Design review of the part built by this model. Coordinates are the model's own, in mm. Face numbers are marked on the shaded views. A direction names the side the tool comes from. Round coordinates to 2 decimals unless told otherwise and drop trailing zeros. Loops run counter-clockwise (first coordinate to the right, second up) from the corner with the lowest first, then second, coordinate; pieces in that order, holes last. Notation, with made-up numbers: M -14.75,85.25 L 22.25,85.25 A32 ccw 22.25,124.25 Z; hole C 16,27.25 d7. An arc over 180 degrees is marked long. Use a Markdown table: item, result.
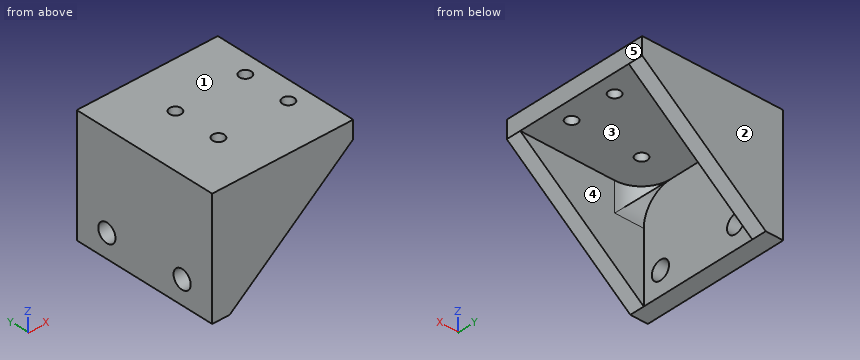
from build123d import *

# Parameters (mm, degrees)
EXTRUDE_1_DEPTH     = 12.6
SKETCH_2_W          = 21.2
SKETCH_2_H          = 20.2
CUT_EXTRUDE_1_DEPTH = 17
SKETCH_3_R          = 1
CUT_EXTRUDE_2_DEPTH = 34.828981658
SKETCH_4_R          = 1.6
CUT_EXTRUDE_3_DEPTH = 32.75216528
FILLET_1_R          = 5
CUT_EXTRUDE_4_DEPTH = 17


with BuildPart() as part:
    # 草图1 → 凸台-拉伸1 (new, symmetric)
    with BuildSketch(Plane(origin=(0, 0, 0), x_dir=(1, 0, 0), z_dir=(0, 1, 0))):
        Polygon((0, 0), (24.2, 0), (24.2, 3), (3, 20), (0, 20), align=None)
    extrude(amount=EXTRUDE_1_DEPTH, both=True)

    # 草图2 → 切除-拉伸1 (cut)
    with BuildSketch(Plane(origin=(0, 0, -20), x_dir=(-1, 0, 0), z_dir=(0, 0, -1))):
        with Locations((-13.6, 0)):
            Rectangle(SKETCH_2_W, SKETCH_2_H)
    extrude(amount=-CUT_EXTRUDE_1_DEPTH, mode=Mode.SUBTRACT)

    # 草图3 → 切除-拉伸2 (cut, through all)
    with BuildSketch(Plane.XY):
        with Locations((21, -4)):
            Circle(SKETCH_3_R)
        with Locations(Location((21, 4, 0), (0, 0, 180))):
            Circle(SKETCH_3_R)
        with Locations((9, 4)):
            Circle(SKETCH_3_R)
        with Locations(Location((9, -4, 0), (0, 0, 180))):
            Circle(SKETCH_3_R)
    extrude(amount=-CUT_EXTRUDE_2_DEPTH, mode=Mode.SUBTRACT)

    # 草图4 → 切除-拉伸3 (cut, through all)
    with BuildSketch(Plane(origin=(3, 0, 0), x_dir=(0, 0, -1), z_dir=(1, 0, 0))):
        with Locations(Location((16, 7, 0), (0, 0, 90))):
            Circle(SKETCH_4_R)
        with Locations(Location((16, -7, 0), (0, 0, 270))):
            Circle(SKETCH_4_R)
    extrude(amount=-CUT_EXTRUDE_3_DEPTH, mode=Mode.SUBTRACT)

    # 圆角1
    fillet_1_edges = [part.edges().sort_by_distance(p)[0] for p in [
        (13.6, -10.1, -3),
        (13.6, 10.1, -3),
    ]]
    fillet(fillet_1_edges, radius=FILLET_1_R)

    # 草图6 → 切除-拉伸4 (cut)
    with BuildSketch(Plane(origin=(0, 0, -20), x_dir=(-1, 0, 0), z_dir=(0, 0, -1))):
        with BuildLine():
            Line((-3, -5.1), (-3, 5.1))
            ThreePointArc((-3, 5.1), (-4.464466094, 8.635533906), (-8, 10.1))
            Line((-8, 10.1), (-24.2, 10.1))
            Line((-24.2, 10.1), (-24.2, -10.1))
            Line((-24.2, -10.1), (-8, -10.1))
            ThreePointArc((-8, -10.1), (-4.464466094, -8.635533906), (-3, -5.1))
        make_face()
    extrude(amount=-CUT_EXTRUDE_4_DEPTH, mode=Mode.SUBTRACT)


solid = part.part
1. Take a section at A-A on y = -4. Give the boundary of the cut face in (x, z), and give its area (3 significant figures).
Check values:
| item | result |
|---|---|
| outline | M 0,-20 L 3,-20 L 3,-3 L 8,-3 L 8,0 L 0,0 Z; M 10,-3 L 20,-3 L 20,0 L 10,0 Z; M 22,-3 L 24.2,-3 L 24.2,0 L 22,0 Z |
| area | 112 mm² |
2. Insertion check: pin 1 (3.5 mm diameter, centred on y = -7, z = -16, fed in from +X); pin 2 (3 mm diameter, centred on x = 9.5, y = 6.5, fed in from -Z). Each pin has a flat end and moves straight along its axis. Give the tip position at first contact, or say it passes through.
Check values:
| item | result |
|---|---|
| pin 1 | stops at x = 3 |
| pin 2 | stops at z = -3 |
3. The part is to be moulded in two halves that separate along Y. For the marked faces 1, 2 and 3, say which applies: pulls with the +Y half, pulls with the -Y half, needs draft (parallel to the pull), parting line crosses it, or undercut.
Check values:
| item | result |
|---|---|
| face 1 | needs draft |
| face 2 | pulls with the +Y half |
| face 3 | undercut |
4. Take a section at C-C on y = 7. Give the boundary of the cut face in (x, z).
Check values:
| item | result |
|---|---|
| outline | M 0,-20 L 3,-20 L 3,-17.6 L 0,-17.6 Z; M 0,-14.4 L 3,-14.4 L 3,-3.38 L 3.38,-3.38 L 3.38,-3 L 24.2,-3 L 24.2,0 L 0,0 Z |
5. Machinability: for the marked faces 4 and 5, which of the approach directions +Z, -Z, +X, -X, +Y, -Y give a long, thin tool a straight path to every point of the face, cutting with its end or side? Answer none if there is none.
Check values:
| item | result |
|---|---|
| face 4 | -Z, +X |
| face 5 | +Z, -Z, +X, +Y, -Y |
6. Take a section at B-B on x = 9. Give the boundary of the cut face in (y, z).
Check values:
| item | result |
|---|---|
| outline | M -12.6,-15.19 L -10.1,-15.19 L -10.1,-3 L -5,-3 L -5,0 L -12.6,0 Z; M -3,-3 L 3,-3 L 3,0 L -3,0 Z; M 5,-3 L 10.1,-3 L 10.1,-15.19 L 12.6,-15.19 L 12.6,0 L 5,0 Z |
7. Wall thickness on line 1 along Y through (x, z) = (21, -2.05); line 2 along Z through (x, y) = (1.4, 7); line 3 along X through (y, z) = (-6.5, -10.5): over which ranges is each line inside the solid? List them lowest first. Write a range as from..to.
Check values:
| item | result |
|---|---|
| line 1 | y = -12.6..-5, -3..3, 5..12.6 |
| line 2 | z = -20..-17.6, -14.4..0 |
| line 3 | x = 0..3 |
8. Take a section at D-D on z = -7.25. Give the boundary of the cut face in (x, y).
Check values:
| item | result |
|---|---|
| outline | M 0,-12.6 L 18.9,-12.6 L 18.9,-10.1 L 8,-10.1 A5 cw 7.25,-10.04 L 3,-10.04 L 3,10.04 L 7.25,10.04 A5 cw 8,10.1 L 18.9,10.1 L 18.9,12.6 L 0,12.6 Z |
